```python
from build123d import *

# Parameters (mm, degrees)
SKETCH1_R           = 1.75
SKETCH1_W           = 7.2
SKETCH1_H           = 5.4
BOSS_EXTRUDE1_DEPTH = 5
FILLET5_RADIUS      = 10
FILLET5_LENGTH      = 5
FILLET2_R           = 5.4
FILLET6_R           = 5.4
SKETCH3_W           = 35
SKETCH3_H           = 20
SKETCH3_W_2         = 23
SKETCH3_H_2         = 13
BOSS_EXTRUDE4_DEPTH = 5.5
SKETCH5_W           = 23
SKETCH5_H           = 13
CUT_EXTRUDE1_DEPTH  = 3.5
CUT_EXTRUDE2_DEPTH  = 76.201396264
FILLET9_R           = 4
SKETCH9_R           = 0.875
CUT_EXTRUDE4_DEPTH  = 7
SKETCH10_W          = 36
SKETCH10_H          = 2.4
BOSS_EXTRUDE5_DEPTH = 30
SKETCH11_R          = 3.25
SKETCH11_R_2        = 0.875
CUT_EXTRUDE5_DEPTH  = 30
FILLET10_R          = 2.5


with BuildPart() as part:
    # Sketch1 → Boss-Extrude1 (new body)
    # profile 1 of 4: a face of its own
    with BuildSketch(Plane(origin=(0, 0, 0), x_dir=(1, 0, 0), z_dir=(0, 1, 0))):
        with BuildLine():
            Line((0, 15), (10, 0))
            Line((10, 0), (26, 0))
            Line((26, 0), (36, 15))
            Line((36, 15), (60, 15))
            Line((60, 15), (60, 25))
            Line((60, 25), (44.5, 25))
            Line((44.5, 25), (44.5, 19.6))
            Line((44.5, 19.6), (37.3, 19.6))
            Line((37.3, 19.6), (26.5, 19.6))
            Line((26.5, 19.6), (26.5, 25))
            Line((26.5, 25), (6.75, 25))
            ThreePointArc((6.75, 25), (5, 23.25), (3.25, 25))
            Line((3.25, 25), (0, 25))
            Line((0, 25), (0, 15))
        make_face()
        with Locations(Location((13, 5, 0), (0, 0, 270))):
            Circle(SKETCH1_R, mode=Mode.SUBTRACT)
        with Locations(Location((23, 5, 0), (0, 0, 270))):
            Circle(SKETCH1_R, mode=Mode.SUBTRACT)
    # profile 2 of 4: a face of its own
    with BuildSketch(Plane(origin=(0, 0, 0), x_dir=(1, 0, 0), z_dir=(0, 1, 0))):
        with BuildLine():
            Line((0, 45), (0, 25))
            Line((0, 25), (3.25, 25))
            ThreePointArc((3.25, 25), (5, 26.75), (6.75, 25))
            Line((6.75, 25), (26.5, 25))
            Line((26.5, 25), (26.5, 30.4))
            Line((26.5, 30.4), (37.3, 30.4))
            Line((37.3, 30.4), (44.5, 30.4))
            Line((44.5, 30.4), (44.5, 25))
            Line((44.5, 25), (60, 25))
            Line((60, 25), (60, 35))
            Line((60, 35), (36, 35))
            Line((36, 35), (36, 45))
            Line((36, 45), (26, 45))
            Line((26, 45), (0, 45))
        make_face()
    # profile 3 of 4: a face of its own
    with BuildSketch(Plane(origin=(0, 0, 0), x_dir=(1, 0, 0), z_dir=(0, 1, 0))):
        with Locations((40.9, 27.7)):
            Rectangle(SKETCH1_W, SKETCH1_H)
    # profile 4 of 4: a face of its own
    with BuildSketch(Plane(origin=(0, 0, 0), x_dir=(1, 0, 0), z_dir=(0, 1, 0))):
        with Locations((40.9, 22.3)):
            Rectangle(SKETCH1_W, SKETCH1_H)
    extrude(amount=BOSS_EXTRUDE1_DEPTH)

    # Fillet5: full round fillet: the end face becomes a half cylinder, R = half its width
    fillet5_face = Plane((60, 2.5, -25), x_dir=(0, -1, 0), z_dir=(1, 0, 0))  # on the end face: x along it, z out of the body
    fillet5_slab = fillet5_face.offset(-FILLET5_RADIUS / 2) * Box(FILLET5_LENGTH, 2 * FILLET5_RADIUS, FILLET5_RADIUS, mode=Mode.PRIVATE)  # the body's end, R deep
    fillet5_round = Plane((50, 2.5, -25), x_dir=(1, 0, 0), z_dir=(0, -1, 0)) * Cylinder(FILLET5_RADIUS, FILLET5_LENGTH, mode=Mode.PRIVATE)  # its axis R under the face
    add(fillet5_slab - fillet5_round, mode=Mode.SUBTRACT)

    # Fillet2
    fillet2_edges = [part.edges().sort_by_distance(p)[0] for p in [
        (26.5, 2.5, -30.4),
        (26.5, 2.5, -19.6),
    ]]
    fillet(fillet2_edges, radius=FILLET2_R - 0.0001)  # a hair under: the kernel refuses the full size

    # Fillet6
    fillet6_edges = [part.edges().sort_by_distance(p)[0] for p in [
        (37.3, 2.5, -19.6),
        (37.3, 2.5, -30.4),
    ]]
    fillet(fillet6_edges, radius=FILLET6_R - 0.0001)  # a hair under: the kernel refuses the full size

    # Sketch3 → Boss-Extrude4 (add)
    with BuildSketch(Plane.XZ):
        with Locations((26.9, -25)):
            Rectangle(SKETCH3_W, SKETCH3_H)
        with Locations((26.9, -25)):
            Rectangle(SKETCH3_W_2, SKETCH3_H_2, mode=Mode.SUBTRACT)
    extrude(amount=BOSS_EXTRUDE4_DEPTH)

    # Sketch5 → Cut-Extrude1 (cut)
    with BuildSketch(Plane.XZ):
        with Locations((26.9, -25)):
            Rectangle(SKETCH5_W, SKETCH5_H)
    extrude(amount=-CUT_EXTRUDE1_DEPTH, mode=Mode.SUBTRACT)

    # Sketch6 → Cut-Extrude2 (cut, through all)
    with BuildSketch(Plane.XZ):
        with BuildLine():
            Line((44.4, -15), (44.4, -35))
            Line((44.4, -35), (50, -35))
            ThreePointArc((50, -35), (60, -25), (50, -15))
            Line((50, -15), (44.4, -15))
        make_face()
    extrude(amount=-CUT_EXTRUDE2_DEPTH, mode=Mode.SUBTRACT)

    # Fillet9
    fillet9_edges = [part.edges().sort_by_distance(p)[0] for p in [
        (44.4, -0.25, -35),
        (44.4, -0.25, -15),
    ]]
    fillet(fillet9_edges, radius=FILLET9_R)

    # Sketch9 → Cut-Extrude4 (cut)
    with BuildSketch(Plane.XZ.offset(5.5)):
        with Locations(Location((13.1, -25, 0), (0, 0, 270))):
            Circle(SKETCH9_R)
        with Locations(Location((40.7, -25, 0), (0, 0, 270))):
            Circle(SKETCH9_R)
    extrude(amount=-CUT_EXTRUDE4_DEPTH, mode=Mode.SUBTRACT)

    # Sketch10 → Boss-Extrude5 (add)
    with BuildSketch(Plane(origin=(0, 5, 0), x_dir=(1, 0, 0), z_dir=(0, 1, 0))):
        with Locations((18, 46.2)):
            Rectangle(SKETCH10_W, SKETCH10_H)
    extrude(amount=-BOSS_EXTRUDE5_DEPTH)

    # Sketch11 → Cut-Extrude5 (cut)
    with BuildSketch(Plane(origin=(0, 0, -47.4), x_dir=(-1, 0, 0), z_dir=(0, 0, -1))):
        with Locations((-18, -10)):
            Circle(SKETCH11_R)
        with Locations((-24.5, -10)):
            Circle(SKETCH11_R_2)
        with Locations((-11.5, -10)):
            Circle(SKETCH11_R_2)
    extrude(amount=-CUT_EXTRUDE5_DEPTH, mode=Mode.SUBTRACT)

    # Fillet10
    fillet10_edges = [part.edges().sort_by_distance(p)[0] for p in [
        (0, -25, -46.2),
        (36, -25, -46.2),
        (18, 5, -47.4),
        (18, 0, -45),
    ]]
    fillet(fillet10_edges, radius=FILLET10_R)


solid = part.part
```
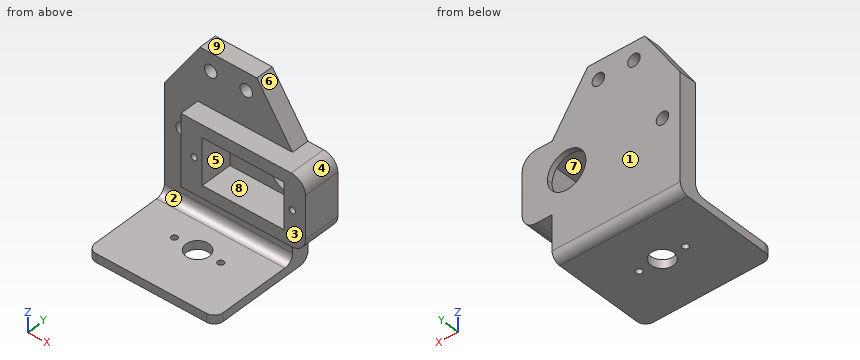
Part model, mm, in its own coordinate system. Face numbers are marked on the shaded views. A direction names the side the tool comes from. Coordinates: 2 decimals unless noted, no trailing zeros. Order: outer loops, then holes, each group sorted by start corner. A loop starts at its lowest first (then second) coordinate and runs counter-clockwise, first axis right, second up. Notation, with made-up numbers: (29.25, 34) - (86.25, 34) arc R21 ccw to (86.25, 54) - close; hole circle Ø4 at (9.5, 25.25). An arc over 180 degrees is marked (long way). Return JSON: item names as keys, results as strings. Group by question number.
Item 1: Cut at B-B (x = 23). List the corners of the cut face in (y, z).
Item 2: Pull direction X, two halves, no side cores. Call the marked faces 6, 7, 8 and 9: pulls with the +X half, pulls with the -X half, needs draft (parallel to the pull), parting line crosses it, or undercut.
Item 3: Cut at C-C (z = -5). List the corners of the cut face in (x, y).
Item 4: Drill centre lines: probe 1 along Z at (x, y) = (17.5, -5); probe 2 along X at (y, z) = (-3.5, -25) (3 decimals); probe 3 along Z at (x, y) = (40.7, -2) (3 decimals). Where is each one in solid material? Low to high. Write a range as from..to.
Item 5: Cut at A-A (y = -1). List the corners of the cut face in (x, z) (3 decimals), plus the area to 3 significant figures.
Item 6: Pin check, flat tips, straight feed: pin 1 (6 mm diameter, centred on x = 31.5, z = -20, fed in from -Y); pin 2 (1.4 mm diameter, centred on x = 13.1, z = -25, fed in from -Y); pin 3 (1.1 mm diameter, centred on x = 24.5, y = -10, fed in from +Z); pin 4 (3 mm diameter, centred on x = 25, y = -2, fed in from +Z). Stop position of each tip, or through.
Item 7: Which spindle directions (+Z, -Z, +X, -X, +Y, -Y) get a long thin tool onto all of the face, cutting with end or side? Do the marked faces 1, 2, 3, 4 and 5. Say none if no direction does.
Item 8: Cut at D-D (x = 5). List the corners of the cut face in (y, z), plus the area to 3 significant figures.
Check values:
{
 "1": {"outline": "(-25, -47.4) - (2.5, -47.4) arc R2.5 ccw to (5, -44.9) - (5, -6.75) - (0, -6.75) - (0, -15) - (-5.5, -15) - (-5.5, -18.5) - (3.5, -18.5) - (3.5, -31.5) - (-5.5, -31.5) - (-5.5, -35) - (0, -35) - (0, -42.5) arc R2.5 cw to (-2.5, -45) - (-25, -45) - close; (0, -3.25) - (5, -3.25) - (5, 0) - (0, 0) - close"},
 "2": {"face 6": "pulls with the +X half", "face 7": "undercut", "face 8": "undercut", "face 9": "needs draft"},
 "3": {"outline": "(6.67, 0) - (11.25, 0) - (11.25, 5) - (6.67, 5) - close; (14.75, 0) - (21.25, 0) - (21.25, 5) - (14.75, 5) - close; (24.75, 0) - (29.33, 0) - (29.33, 5) - (24.75, 5) - close"},
 "4": {"probe 1": "z = -47.4..-45, -35..-31.5, -18.5..-15", "probe 2": "x = 9.4..12.225, 13.975..15.4, 38.4..39.825, 41.575..44.4", "probe 3": "z = -34.989..-25.875, -24.125..-15.011"},
 "5": {"outline": "(0, -47.4) - (36, -47.4) - (36, -44.5) - (0, -44.5) - close; (9.4, -35) - (40.4, -35) arc R4 ccw to (44.4, -31) - (44.4, -19) arc R4 ccw to (40.4, -15) - (9.4, -15) - close; hole circle Ø1.75 at (13.1, -25); hole (15.4, -31.5) - (38.4, -31.5) - (38.4, -18.5) - (15.4, -18.5) - close; hole circle Ø1.75 at (40.7, -25)", "area": "494 mm2"},
 "6": {"pin 1": "stops at y = -5.5", "pin 2": "stops at y = 1.5", "pin 3": "passes through", "pin 4": "stops at z = -15"},
 "7": {"face 1": "+Z, -Z, +X, -X, +Y", "face 2": "+X, -X, -Y", "face 3": "+Z, +X, -X, -Y", "face 4": "+Z, +X, +Y, -Y", "face 5": "-Y"},
 "8": {"outline": "(-25, -47.4) - (2.5, -47.4) arc R2.5 ccw to (5, -44.9) - (5, -26.75) - (0, -26.75) - (0, -42.5) arc R2.5 cw to (-2.5, -45) - (-25, -45) - close; (0, -23.25) - (5, -23.25) - (5, -7.5) - (0, -7.5) - close", "area": "242 mm2"}
}
